Source: CAD feature listing. Evaluate the final solid. Frame: model axes, mm. Face numbers are marked on the shaded views. Round coordinates to 2 decimals unless told otherwise and drop trailing zeros. Loops run counter-clockwise (first coordinate to the right, second up) from the corner with the lowest first, then second, coordinate; pieces in that order, holes last. Notation, with made-up numbers: (-5, 23.25) - (46, 23.25) arc R15 cw to (46, 29.25) - close; hole circle Ø3 at (43, 57.25). An arc over 180 degrees is marked (long way). Write item = value, one per line. Start each with the question number.
from build123d import *

# Parameters (mm, degrees)
F0_W     = 76.2
F0_H     = 127
F1_DEPTH = 127
F2_T     = -2.54
F3_W     = 63.5
F3_H     = 114.3
F4_DEPTH = 76.2
F5_R     = 5.9944


with BuildPart() as f1:
    # F0 (on Front) → F1 (new body)
    with BuildSketch(Plane.XZ):
        with Locations((-38.1, -2.7002265453)):
            Rectangle(F0_W, F0_H)
    extrude(amount=-F1_DEPTH)

    # F2 (hollow: no face is removed)
    offset(amount=F2_T, mode=Mode.SUBTRACT)

    # F3 (on face) → F4 (cut)
    with BuildSketch(Plane.XZ):
        with Locations((-38.1208891869, -3.2391424835)):
            Rectangle(F3_W, F3_H)
    extrude(amount=-F4_DEPTH, mode=Mode.SUBTRACT)

    # F5
    f5_edges = [f1.edges().sort_by_distance(p)[0] for p in [
        (0, 63.5, 60.799773),
        (-38.1, 0, 60.799773),
        (0, 0, -2.700227),
        (-76.2, 63.5, 60.799773),
        (-76.2, 63.5, -66.200227),
        (-76.2, 0, -2.700227),
        (-76.2, 127, -2.700227),
        (-38.1, 127, 60.799773),
    ]]
    fillet(f5_edges, radius=F5_R)


solid = f1.part
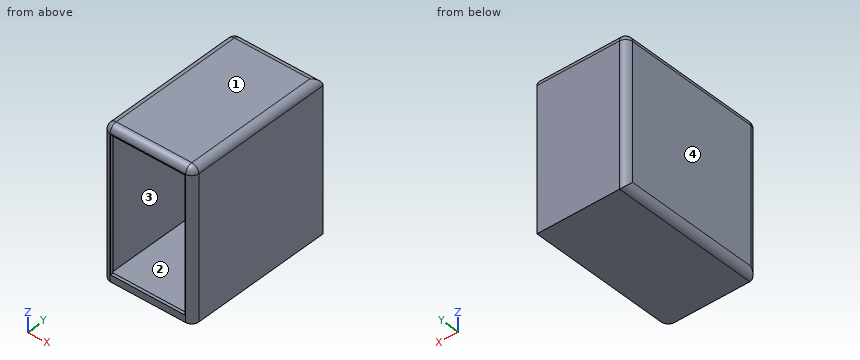
(1) Mould query, pull axis X, two halves, no side actions, for the marked faces 1, 2, 3 and 4. Classes: +X half, -X half, draft (parallel to the pull), parting line (faces both ways), or undercut.
(2) Cut plane C-C (z = 4). Output: boundary loops of the cut face in (x, y).
(3) Pin query (flat end, axial travel): P1, Ø0.8, axis at y = 2, z = 8.5, coming from the +X side; P2, Ø3, axis at y = 1, z = -31.5, coming from the -X side; P3, Ø2, axis at x = -22, z = -41.5, coming from the -Y side. Return the tip coordinate at first contact, or that it passes through.
(4) Cut plane B-B (x = -67). Output: boundary loops of the cut face in (y, z), and give its area (3 significant figures).
(5) Cut plane A-A (y = 75). Output: boundary loops of the cut face in (x, z).
(6) Material intervals for line 1 along X through (y, z) = (9.5, -41); line 2 along Z through (x, y) = (-18.5, 89); line 3 along Y through (x, z) = (-49, 19), sorted ascending. Write a range as from..to.
Solution:
q1.face_1 = draft
q1.face_2 = undercut
q1.face_3 = undercut
q1.face_4 = -X half
q2.outline = (-76.2, 5.99) arc R5.99 ccw to (-70.21, 0) - (-69.87, 0) - (-69.87, 2.54) - (-73.66, 2.54) - (-73.66, 124.46) - (-2.54, 124.46) - (-2.54, 2.54) - (-6.37, 2.54) - (-6.37, 0) - (-5.99, 0) arc R5.99 ccw to (0, 5.99) - (0, 127) - (-70.21, 127) arc R5.99 ccw to (-76.2, 121.01) - close
q3.P1 = -1.2
q3.P2 = -75.08
q3.P3 = 124.46
q4.outline = (0, -66.2) - (127, -66.2) - (127, 54.81) arc R5.99 ccw to (121.01, 60.8) - (5.99, 60.8) arc R5.99 ccw to (0, 54.81) - (0, 53.91) - (2.54, 53.91) - (2.54, 58.26) - (124.46, 58.26) - (124.46, -63.66) - (2.54, -63.66) - (2.54, -60.39) - (0, -60.39) - close
q4.area = 959 mm^2
q5.outline = (-76.2, -60.21) arc R5.99 ccw to (-70.21, -66.2) - (0, -66.2) - (0, 54.81) arc R5.99 ccw to (-5.99, 60.8) - (-70.21, 60.8) arc R5.99 ccw to (-76.2, 54.81) - close; hole (-73.66, -63.66) - (-2.54, -63.66) - (-2.54, 58.26) - (-73.66, 58.26) - close
q6.line_1 = -76.2..-73.66, -2.54..0
q6.line_2 = -66.2..-63.66, 58.26..60.8
q6.line_3 = 124.46..127
